For this review, take the finished solid that the model builds, in its own axes (mm). A direction names the side the tool comes from. Round coordinates to 2 decimals unless told otherwise and drop trailing zeros. Write each loop counter-clockwise with the first axis right and the second up, starting at its lowest first coordinate (ties: lowest second). Pieces come first, ordered by that corner, then holes. Notation, with made-up numbers: (43, 33.25) -> (87, 33.25) arc R32 ccw to (87, 71.25) -> close; hole circle Ø9 at (61.25, 32.25). An arc over 180 degrees is marked (long way). Answer as CSV lines item,"result". Start each with the question number.
Item 1: Take a section at C-C on z = -35.5. Give the boundary of the cut face in (x, y).
Item 2: Take a section at D-D on x = -247. Give the boundary of the cut face in (y, z), then the cut area to 3 significant figures.
Item 3: For pin 1 Ø8 at (y, z) = (-3.5, 392) entering from +X; pin 2 Ø12 at (x, y) = (-334.5, -6.5) entering from -Z; pin 3 Ø3 at (x, y) = (-326.5, -15.5) entering from +Z, all flat-tipped, find the tip position at first contact; note any pin that passes through.
Item 4: Wall thickness on probe 1 along Z at (x, y) = (-323, -21.75); probe 2 along Z at (x, y) = (-380, -12.25); probe 3 along X at (y, z) = (-8, 375.5): over which ranges is each line inside the solid? List them lowest first. Write a range as from..to.
Item 5: Take a section at A-A on y = -4.5. Give the boundary of the cut face in (x, z).
Item 6: Take a section at B-B on x = -356.5. Give the boundary of the cut face in (y, z).
Item 7: Machinability: for faces 1 (the flat face through (-383.277, -12.325, -9.385)), 2 (the flat face through (-440, -12, 455.703)), which of the approach directions +Z, -Z, +X, -X, +Y, -Y give a long, thin tool a straight path to every point of the face, cutting with its end or side? Answer none if there is none.
```python
from build123d import *

# Parameters (mm, degrees)
F2_DEPTH = 25


with BuildPart() as f2:
    # F1 (on face) → F2 (new body)
    with BuildSketch(Plane.XZ):
        with BuildLine():
            Line((-297.94293, 60.56272), (-287.904638, 78.745993))
            Line((-287.904638, 78.745993), (-264.119575, 121.830047))
            ThreePointArc((-264.119575, 121.830047), (-251.165034, 135.11697), (-233.238659, 139.913584))
            Line((-233.238659, 139.913584), (-213.697833, 139.779545))
            ThreePointArc((-213.697833, 139.779545), (-221.348908, 163.277257), (-218.880566, 187.865643))
            Line((-218.880566, 187.865643), (-260.360033, 187.611007))
            ThreePointArc((-260.360033, 187.611007), (-279.922741, 193.444261), (-292.903603, 209.199373))
            Line((-292.903603, 209.199373), (-363.591224, 344.828208))
            Line((-363.591224, 344.828208), (-381.832675, 379.828208))
            Line((-381.832675, 379.828208), (-421.377269, 455.702698))
            Line((-421.377269, 455.702698), (-458.70873, 455.702698))
            Line((-458.70873, 455.702698), (-318.796581, 187.252275))
            Line((-318.796581, 187.252275), (-310.806441, 171.921537))
            ThreePointArc((-310.806441, 171.921537), (-307.018527, 159.236472), (-308.213044, 146.051924))
            Line((-308.213044, 146.051924), (-311.319953, 135.27254))
            Line((-311.319953, 135.27254), (-457.277019, -158.149611))
            Line((-457.277019, -158.149611), (-418.685669, -158.149611))
            Line((-418.685669, -158.149611), (-297.94293, 60.56272))
        make_face()
    extrude(amount=F2_DEPTH)


solid = f2.part
```
Output values:
1,outline,"(-396.27, -25) -> (-350.98, -25) -> (-350.98, 0) -> (-396.27, 0) -> close"
2,outline,"(-25, 137.2) -> (0, 137.2) -> (0, 187.69) -> (-25, 187.69) -> close"
2,area,"1,260 mm^2"
3,pin 1,"stops at x = -386.09"
3,pin 2,"stops at z = -16.52"
3,pin 3,"stops at z = 276.54"
4,probe 1,"z = 15.17..111.79, 195.32..266.95"
4,probe 2,"z = -88.07..-2.8, 304.68..376.31"
4,probe 3,"x = -416.91..-379.58"
5,outline,"(-458.71, 455.7) -> (-310.81, 171.92) arc R35 cw to (-308.21, 146.05) -> (-311.32, 135.27) -> (-457.28, -158.15) -> (-418.69, -158.15) -> (-264.12, 121.83) arc R35 cw to (-233.24, 139.91) -> (-213.7, 139.78) arc R60 cw to (-218.88, 187.87) -> (-260.36, 187.61) arc R35 cw to (-292.9, 209.2) -> (-421.38, 455.7) -> close"
6,outline,"(-25, -45.51) -> (0, -45.51) -> (0, 44.45) -> (-25, 44.45) -> close; (-25, 259.59) -> (0, 259.59) -> (0, 331.22) -> (-25, 331.22) -> close"
7,face 1,"-X, +Y, -Y"
7,face 2,"+Z, +X, -X, +Y, -Y"
